Read the model definition and answer for the solid it produces. Units are mm, in the model's axes. Face numbers are marked on the shaded views. A direction names the side the tool comes from. Round coordinates to 2 decimals unless told otherwise and drop trailing zeros. Loops run counter-clockwise (first coordinate to the right, second up) from the corner with the lowest first, then second, coordinate; pieces in that order, holes last. Notation, with made-up numbers: (-6, -12) - (26, -12) arc R11 ccw to (26, 8) - close; hole circle Ø3 at (5.5, 41.25). An arc over 180 degrees is marked (long way). Answer as CSV lines item,"result".
```python
from build123d import *

# Parameters (mm, degrees)
F0_W           = 70
F0_H           = 60
F0_W_2         = 19.25
F0_H_2         = 32
F1_DEPTH       = 3
F2_DEPTH       = 32
F4_D           = 6.3
F5_R           = 15
F6_SIZE        = 20
F7_D           = 3.5
F7_CSINK_D     = 6.5
F7_CSINK_ANGLE = 82
F8_SIZE        = 0.3


# Not quite as in the source:
# - a feature names something its author has since deleted; it is built from what else it names


with BuildPart() as f1:
    # F0 (on Top) → F1 (new body)
    with BuildSketch(Plane.XY):
        Rectangle(F0_W, F0_H)
        with Locations((-11.375, 0)):
            Rectangle(F0_W_2, F0_H_2, mode=Mode.SUBTRACT)
        with Locations((11.375, 0)):
            Rectangle(F0_W_2, F0_H_2, mode=Mode.SUBTRACT)
        with Locations((11.375, 0)):
            Rectangle(F0_W_2, F0_H_2)
        with Locations((-11.375, 0)):
            Rectangle(F0_W_2, F0_H_2)
    extrude(amount=F1_DEPTH)

    # F0 (on Top) → F2 (join)
    with BuildSketch(Plane.XY):
        with Locations((-11.375, 0)):
            Rectangle(F0_W_2, F0_H_2)
        with Locations((11.375, 0)):
            Rectangle(F0_W_2, F0_H_2)
    extrude(amount=-F2_DEPTH)

    # F4 (through all)
    with Locations(Plane.YZ.offset(21)):
        with Locations((0, -16)):
            Hole(F4_D / 2)

    # F5
    f5_edges = [f1.edges().sort_by_distance(p)[0] for p in [
        (11.375, 16, -32),
        (11.375, -16, -32),
        (-11.375, -16, -32),
        (-11.375, 16, -32),
    ]]
    fillet(f5_edges, radius=F5_R)

    # F6
    f6_edges = [f1.edges().sort_by_distance(p)[0] for p in [
        (-35, 30, 1.5),
        (-35, -30, 1.5),
        (35, -30, 1.5),
        (35, 30, 1.5),
    ]]
    chamfer(f6_edges, length=F6_SIZE)

    # F7 (through all)
    with Locations(Plane(origin=(0, 0, 0), x_dir=(1, 0, 0), z_dir=(0, 0, -1))):
        with Locations((-11.375, -23), (11.375, -23), (28, -8), (28, 8), (11.375, 23), (-11.375, 23), (-27.5449063629, 8), (-27.5449063629, -8)):
            CounterSinkHole(F7_D / 2, F7_CSINK_D / 2, counter_sink_angle=F7_CSINK_ANGLE)

    # F8
    f8_edges = [f1.edges().sort_by_distance(p)[0] for p in [
        (1.75, -16, -8.5),
        (21, -16, -8.5),
        (0, -30, 0),
        (35, 0, 0),
        (0, -30, 3),
        (35, 0, 3),
        (0, 30, 3),
        (0, 30, 0),
        (-35, 0, 3),
        (-35, 0, 0),
        (-25, -20, 0),
        (-25, -20, 3),
        (-25, 20, 0),
        (-25, 20, 3),
        (25, 20, 3),
        (25, 20, 0),
        (25, -20, 3),
        (25, -20, 0),
        (-21, 16, -8.5),
        (-21, 11.606602, -27.606602),
        (-21, 0, -32),
        (-21, -16, -8.5),
        (-21, -11.606602, -27.606602),
        (-21, -3.15, -16),
        (-1.75, 16, -8.5),
        (-1.75, -16, -8.5),
        (-1.75, -11.606602, -27.606602),
        (-1.75, 0, -32),
        (-1.75, 11.606602, -27.606602),
        (-1.75, -3.15, -16),
        (1.75, 16, -8.5),
        (1.75, 11.606602, -27.606602),
        (1.75, 0, -32),
        (1.75, -11.606602, -27.606602),
        (1.75, -3.15, -16),
        (21, -11.606602, -27.606602),
        (21, 0, -32),
        (21, 16, -8.5),
        (21, 11.606602, -27.606602),
        (21, -3.15, -16),
    ]]
    chamfer(f8_edges, length=F8_SIZE)


solid = f1.part
```
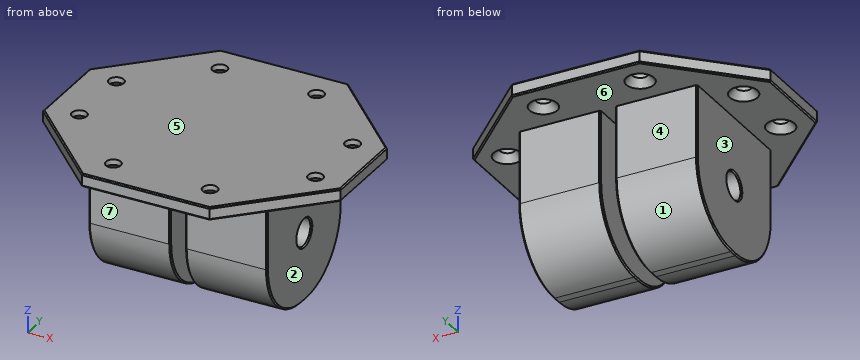
1) The mould has two halves that part along X. Classify the marked faces 1, 2 and 3: pulls with the +X half, pulls with the -X half, needs draft (parallel to the pull), parting line crosses it, or undercut.
Entries:
face 1,"needs draft"
face 2,"pulls with the +X half"
face 3,"pulls with the -X half"
2) A cutting plane is placed at C-C, the plane z = -16. Count the separate pieces of the cut face and the enclosed holes in it, plus the area to 3 significant figures.
Entries:
separate pieces,"4"
enclosed holes,"0"
area,"989 mm^2"
3) A cutting plane is placed at B-B, the plane x = -5.5. Determine the outline of the cut face in (y, z), plus the area to 3 significant figures.
Entries:
outline,"(-30, 0.3) - (-29.7, 0) - (-16, 0) - (-16, -17) arc R15 ccw to (-1, -32) - (1, -32) arc R15 ccw to (16, -17) - (16, 0) - (29.7, 0) - (30, 0.3) - (30, 2.7) - (29.7, 3) - (-29.7, 3) - (-30, 2.7) - close; hole circle Ø6.3 at (0, -16)"
area,"1,080 mm^2"
4) Find the intervals of material crossed by line 1 (X direction, y = -8, z = 2); line 2 (X direction, y = -10, z = -9.5), in increasing order.
Entries:
line 1,"x = -35 to -29.29, -25.79 to 26.25, 29.75 to 35"
line 2,"x = -21 to -1.75, 1.75 to 21"
5) Each of these flat-tipped pins is pushed along its axis until it touches: P1, Ø3, axis at x = -27.54, y = 8, coming from the +Z side; P2, Ø5, axis at x = -12.5, z = -10.5, coming from the +Y side; P3, Ø4, axis at x = 11.375, y = -23, coming from the -Z side; P4, Ø2, axis at y = 7, z = -6, coming from the +X side. Where does it stop, or does it pass through?
Entries:
P1,"passes through"
P2,"stops at y = 16"
P3,"stops at z = 1.44"
P4,"stops at x = 21"
6) A tool of negligible diameter and unlimited length cuts with its end or side. For the marked faces 4, 5, 6 and 7, from which of +Z, -Z, +X, -X, +Y, -Y can it reach the whole face along a straight path? Write none if from no direction.
Entries:
face 4,"-Z, +X, -X, +Y"
face 5,"+Z, +X, -X, +Y, -Y"
face 6,"-Z"
face 7,"-Z, +X, -X, -Y"
7) A cutting plane is placed at A-A, the plane z = -5. Determine the outline of the cut face in (x, y), plus the area to 3 significant figures.
Entries:
outline,"(-21, -15.7) - (-20.7, -16) - (-2.05, -16) - (-1.75, -15.7) - (-1.75, 15.7) - (-2.05, 16) - (-20.7, 16) - (-21, 15.7) - close; (1.75, -15.7) - (2.05, -16) - (20.7, -16) - (21, -15.7) - (21, 15.7) - (20.7, 16) - (2.05, 16) - (1.75, 15.7) - close"
area,"1,230 mm^2"
8) A cutting plane is placed at D-D, the plane x = 28. Determine the outline of the cut face in (y, z), plus the area to 3 significant figures.
Entries:
outline,"(-17, 0.3) - (-16.58, 0) - (-11.25, 0) - (-9.75, 1.73) - (-9.75, 3) - (-16.58, 3) - (-17, 2.7) - close; (-6.25, 1.73) - (-4.75, 0) - (4.75, 0) - (6.25, 1.73) - (6.25, 3) - (-6.25, 3) - close; (9.75, 1.73) - (11.25, 0) - (16.58, 0) - (17, 0.3) - (17, 2.7) - (16.58, 3) - (9.75, 3) - close"
area,"75.6 mm^2"
